```python
from build123d import *

# Parameters (mm, degrees)
BOSS_EXTRUDE1_DEPTH = 0.5
SKETCH2_W           = 2.54
SKETCH2_H           = 2.54
BOSS_EXTRUDE2_DEPTH = 3
SKETCH3_OUTSIDE_W   = 12.904
SKETCH3_OUTSIDE_H   = 6.694
SKETCH3_OUTSIDE_R   = 0.25
CUT_EXTRUDE1_DEPTH  = 0.5


with BuildPart() as part:
    # Sketch1 → Boss-Extrude1 (new body)
    with BuildSketch(Plane(origin=(0, 0, 0), x_dir=(1, 0, 0), z_dir=(0, 1, 0))):
        Polygon((0, 0), (4.72, 0), (4.72, 3.649976519), (4.72, 8.75), (4.22, 8.75), (4.22, 0.5), (0, 0.5), align=None)
    extrude(amount=BOSS_EXTRUDE1_DEPTH)

    # Sketch2 → Boss-Extrude2 (add)
    with BuildSketch(Plane(origin=(0, 0, -4.75), x_dir=(-1, 0, 0), z_dir=(0, 0, -1))):
        with Locations((-4.47, 0.25)):
            Rectangle(SKETCH2_W, SKETCH2_H)
    extrude(amount=-BOSS_EXTRUDE2_DEPTH)

    # Sketch3 outside → Cut-Extrude1 (cut)
    with BuildSketch(Plane.ZY):
        with Locations((-4.375, 0.25)):
            Rectangle(SKETCH3_OUTSIDE_W, SKETCH3_OUTSIDE_H)
        with Locations((-0.25, 0.25)):
            Circle(SKETCH3_OUTSIDE_R, mode=Mode.SUBTRACT)
    extrude(amount=-CUT_EXTRUDE1_DEPTH, mode=Mode.SUBTRACT)


solid = part.part
```
Verification items for the finished model (mm, model axes). A direction names the side the tool comes from. Give positions to 0.01 mm unless a question says otherwise; leave off trailing zeros. Loops run counter-clockwise (first coordinate to the right, second up) from the corner with the lowest first, then second, coordinate; pieces in that order, holes last.
1. Thickness scan on line 1 (Y direction, x = 0.85, z = -0.25); line 2 (X direction, y = 0.4, z = -7.25); line 3 (Z direction, x = 4, y = -0.05). Record the ranges inside material, lowest first.
2. Set-up check for faces 1 (the flat face through (4, -1.02, -3)), 2 (the flat face through (3, 0, -0.3)), 3 (the flat face through (3, 0.5, -0.3)): record each of +Z, -Z, +X, -X, +Y, -Y from which the full face is reachable in a straight line by a thin tool's end or side.
3. Go/stop test with flat-tipped pins: pin 1 Ø1 at (x, y) = (5, 0) entering from +Z; pin 2 Ø0.8 at (y, z) = (1, -3) entering from -X; pin 3 Ø1.5 at (x, y) = (2.5, 0.5) entering from -Z; pin 4 Ø1.5 at (x, y) = (1.5, 0) entering from -Z. Record where each tip stops, or that it passes through.
4. Section check B-B, the plane y = 0.6. Enter the section's corners in (x, z).
5. Section check A-A, the plane x = 3.3. Enter the section's corners in (y, z), then the cut area to 3 significant figures.
6. Section check C-C, the plane z = -4.25. Enter the section's corners in (x, y), then the cut area to 3 significant figures.
Geometry says:
1. line 1: y = 0 to 0.5
1. line 2: x = 4.22 to 4.72
1. line 3: z = -4.75 to -1.75
2. face 1: +Z, -Z, +X, -X, -Y
2. face 2: +Z, +X, -X, -Y
2. face 3: +Z, +X, -X, +Y
3. pin 1: stops at z = 0
3. pin 2: stops at x = 3.2
3. pin 3: stops at z = -4.75
3. pin 4: stops at z = -0.5
4. outline: (3.2, -4.75) - (5.74, -4.75) - (5.74, -1.75) - (3.2, -1.75) - close
5. outline: (-1.02, -4.75) - (1.52, -4.75) - (1.52, -1.75) - (-1.02, -1.75) - close; (0, -0.5) - (0.5, -0.5) - (0.5, 0) - (0, 0) - close
5. area: 7.87 mm2
6. outline: (3.2, -1.02) - (5.74, -1.02) - (5.74, 1.52) - (3.2, 1.52) - close
6. area: 6.45 mm2
